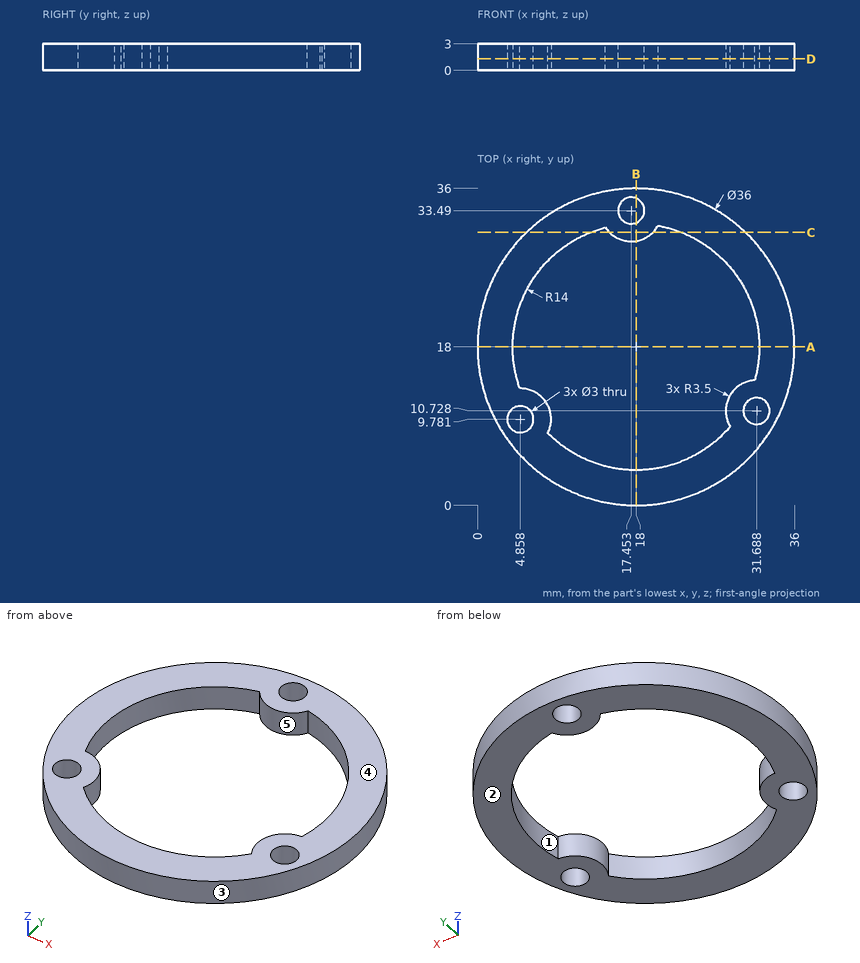
Could you check a few things on this drawing? It's one solid part, dimensions in mm from its lowest x, y, z. A direction names the side the tool comes from. Coordinates: 2 decimals unless noted, no trailing zeros. Order: outer loops, then holes, each group sorted by start corner. A loop starts at its lowest first (then second) coordinate and runs counter-clockwise, first axis right, second up. Notation, with made-up numbers: (-5.5, 81) -> (8.5, 81) arc R17 ccw to (8.5, 93) -> close; hole circle Ø9 at (-35, 12). An arc over 180 degrees is marked (long way). One line per item, written item: value. Start each with the question number.
1) Imagine slicing it at C-C on y = 31. List the corners of the cut face in (x, z) for me.
2) Imagine slicing it at D-D on z = 1.3. List the corners of the cut face in (x, y) for me (1 decimal).
3) Imagine slicing it at B-B on x = 18. List the corners of the cut face in (y, z) for me.
4) Which directions (+Z, -Z, +X, -X, +Y, -Y) give clear straight access to the entire face, cutting with the end or side of a thin tool? Please do the marked faces 4 and 5.
5) Imagine slicing it at A-A on y = 18. List the corners of the cut face in (x, z) for me, plus the area to 3 significant figures.
6) I'm going to push flat-ended pins straight in: pin 1 (2.5 mm diameter, centred on x = 31.69, y = 10.73, fed in from +Z); pin 2 (1 mm diameter, centred on y = 15.5, z = 0.5, fed in from +X). Where does each tip first touch, or does it pass through?
7) If I drill on L1, parallel to X at y = 9, z = 2 (1 decimal); L2, parallel to Y at x = 12.5, z = 2.35 (1 decimal); L3, parallel to Y at x = 14.5, z = 1.85 (1 decimal), over which ranges is the centre line in solid material (lowest first)? Write a range as [from, to].
8) We'd pull the mould along Y, two halves only. Please class the marked faces 1, 2 and 3: +Y half, -Y half, draft (parallel to the pull), parting line (faces both ways), or undercut.
Answer list:
1. outline: (5.55, 0) -> (12.8, 0) -> (12.8, 3) -> (5.55, 3) -> close; (14.99, 0) -> (19.91, 0) -> (19.91, 3) -> (14.99, 3) -> close; (23.2, 0) -> (30.45, 0) -> (30.45, 3) -> (23.2, 3) -> close
2. outline: circle Ø36 at (18, 18); hole circle Ø3 at (4.9, 9.8); hole (4.8, 13.3) arc R3.5 cw to (8, 8.2) arc R14 ccw to (28.7, 8.9) arc R3.5 cw to (31.5, 14.2) arc R14 ccw to (20.5, 31.8) arc R3.5 cw to (14.5, 31.6) arc R14 ccw to start; hole circle Ø3 at (17.5, 33.5); hole circle Ø3 at (31.7, 10.7)
3. outline: (0, 0) -> (4, 0) -> (4, 3) -> (0, 3) -> close; (30.03, 0) -> (32.09, 0) -> (32.09, 3) -> (30.03, 3) -> close; (34.89, 0) -> (36, 0) -> (36, 3) -> (34.89, 3) -> close
4. face 4: +Z, +X, -X, +Y, -Y
4. face 5: +Z, -Z
5. outline: (0, 0) -> (4, 0) -> (4, 3) -> (0, 3) -> close; (32, 0) -> (36, 0) -> (36, 3) -> (32, 3) -> close
5. area: 24.0 mm2
6. pin 1: passes through
6. pin 2: stops at x = 35.89
7. L1: x = [2.4, 3.6], [6.1, 8.3], [28.6, 33.6]
7. L2: y = [0.9, 5.1], [30.9, 35.1]
7. L3: y = [0.3, 4.4], [31.6, 35.7]
8. face 1: undercut
8. face 2: draft
8. face 3: parting line
